Here's how the part is built. I have some questions about the finished solid (model axes, mm). A direction names the side the tool comes from. Coordinates: 2 decimals unless noted, no trailing zeros. Loops run counter-clockwise (first coordinate to the right, second up) from the corner with the lowest first, then second, coordinate; pieces in that order, holes last.
from build123d import *

# Parameters (mm, degrees)
SKETCH1_R           = 6
BOSS_EXTRUDE2_DEPTH = 10


with BuildPart() as part:
    # Sketch1 → Boss-Extrude2 (new, symmetric)
    with BuildSketch(Plane.XY):
        with BuildLine():
            ThreePointArc((27.928480088, -14), (17.026317786, -9.710800875), (11.969348609, 0.857142857))
            ThreePointArc((11.969348609, 0.857142857), (-0.428845364, 11.992334704), (-12, 0))
            Line((-12, 0), (-12, -80))
            ThreePointArc((-12, -80), (-6.142135624, -94.142135624), (8, -100))
            Line((8, -100), (57.751288694, -100))
            ThreePointArc((57.751288694, -100), (65.751288694, -102.143593539), (71.607695155, -108))
            ThreePointArc((71.607695155, -108), (83.566314307, -113.897338336), (93.591109915, -105.105828541))
            Line((93.591109915, -105.105828541), (111.256852168, -39.176380902))
            ThreePointArc((111.256852168, -39.176380902), (107.805402448, -21.82477142), (91.938335642, -14))
            Line((91.938335642, -14), (27.928480088, -14))
        make_face()
        with Locations((82, -102)):
            Circle(SKETCH1_R, mode=Mode.SUBTRACT)
        with BuildLine():
            Line((-5, -80), (-5, -34))
            ThreePointArc((-5, -34), (-1.192388155, -24.807611845), (8, -21))
            Line((8, -21), (91.938335642, -21))
            ThreePointArc((91.938335642, -21), (102.251929066, -26.086101423), (104.495371384, -37.364647586))
            Line((104.495371384, -37.364647586), (94.75149343, -73.729295173))
            ThreePointArc((94.75149343, -73.729295173), (85.465219101, -87.627186848), (69.637421946, -93))
            Line((69.637421946, -93), (8, -93))
            ThreePointArc((8, -93), (-1.192388155, -89.192388155), (-5, -80))
        make_face(mode=Mode.SUBTRACT)
        Circle(SKETCH1_R, mode=Mode.SUBTRACT)
    extrude(amount=BOSS_EXTRUDE2_DEPTH, both=True)


solid = part.part
Q1. Will these pins go through, and if not, where does the flat tip stop? P1, Ø2, axis at x = 10.5, z = -5, coming from the +Y side; P2, Ø2, axis at y = -60, z = 5.5, coming from the +X side; P3, Ø11, axis at x = 0, y = 0, coming from the -Z side; P4, Ø10, axis at x = 57.5, z = -7, coming from the +Y side.
Q2. We'd pull the mould along X, two halves only. Please class faces 4 (the cylindrical face through (65.65, -102.085, 0.14)), 5 (the cylindrical face through (77.58, -97.94, -0.14)), 6 (the cylindrical face through (107.96, -22.03, 0.14)): pulls with the +X half, pulls with the -X half, needs draft (parallel to the pull), parting line crosses it, or undercut.
Q3. Suppose I cut it at D-D on x = 15. Write out the boundary of the cut face in (y, z), and give its area (3 significant figures).
Q4. Suppose I cut it at C-C on z = 5.75. Write out the boundary of the cut face in (x, y), and give its area (3 significant figures).
Q5. Suppose I cut it at A-A on x = 81.5. Write out the boundary of the cut face in (y, z).
Q6. Please list where these lines run through material, in increasing order: probe 1 along Y at (x, z) = (82, 4.5); probe 2 along Y at (x, z) = (4, -4.5); probe 3 along Y at (x, z) = (35.5, 4.75).
Q7. For faces 1 (the cylindrical face through (83.37, -113.92, 0.14)), 2 (the cylindrical face through (85.654, -87.481, 0.14)), 3 (the flat face through (33, -100, 0)), which set-ups out of +Z, -Z, +X, -X, +Y, -Y let a thin tool reach every point of the face, with its end or its side?
Q8. Suppose I cut it at B-B on y = 3. Write out the boundary of the cut face in (x, z).
Check values:
1. P1: stops at y = 7.33
1. P2: stops at x = 105.95
1. P3: passes through
1. P4: stops at y = -14
2. face 4: pulls with the -X half
2. face 5: undercut
2. face 6: pulls with the +X half
3. outline: (-100, -10) - (-93, -10) - (-93, 10) - (-100, 10) - close; (-21, -10) - (-7.43, -10) - (-7.43, 10) - (-21, 10) - close
3. area: 411 mm2
4. outline: (-12, -80) arc R20 ccw to (8, -100) - (57.75, -100) arc R16 cw to (71.61, -108) arc R12 ccw to (93.59, -105.11) - (111.26, -39.18) arc R20 ccw to (91.94, -14) - (27.93, -14) arc R16 cw to (11.97, 0.86) arc R12 ccw to (-12, 0) - close; hole circle Ø12 at (0, 0); hole (-5, -80) arc R13 ccw to (8, -93) - (69.64, -93) arc R26 ccw to (94.75, -73.73) - (104.5, -37.36) arc R13 ccw to (91.94, -21) - (8, -21) arc R13 ccw to (-5, -34) - close; hole circle Ø12 at (82, -102)
4. area: 3,350 mm2
5. outline: (-113.99, -10) - (-107.98, -10) - (-107.98, 10) - (-113.99, 10) - close; (-96.02, -10) - (-90.14, -10) - (-90.14, 10) - (-96.02, 10) - close; (-21, -10) - (-14, -10) - (-14, 10) - (-21, 10) - close
6. probe 1: y = -114 to -108, -96 to -89.87, -21 to -14
6. probe 2: y = -99.6 to -92.37, -21.63 to -4.47, 4.47 to 11.31
6. probe 3: y = -100 to -93, -21 to -14
7. face 1: +Z, -Z, -Y
7. face 2: +Z, -Z
7. face 3: +Z, -Z, -X, -Y
8. outline: (-11.62, -10) - (-5.2, -10) - (-5.2, 10) - (-11.62, 10) - close; (5.2, -10) - (11.62, -10) - (11.62, 10) - (5.2, 10) - close
